```python
from build123d import *

# Parameters (mm, degrees)
F0_R     = 775
F0_R_2   = 16.5
F0_R_3   = 475
F1_DEPTH = 160
F3_DEPTH = 160


with BuildPart() as f1:
    # F0 (on Front) → F1 (new body)
    with BuildSketch(Plane.XZ):
        Circle(F0_R)
        with Locations((-389.681126, -488.644677)):
            Circle(F0_R_2, mode=Mode.SUBTRACT)
        with Locations((-488.644677, -389.681126)):
            Circle(F0_R_2, mode=Mode.SUBTRACT)
        with Locations((-441.941738, -441.941738)):
            Circle(F0_R_2, mode=Mode.SUBTRACT)
        with Locations((-206.424414, -589.927081)):
            Circle(F0_R_2, mode=Mode.SUBTRACT)
        with Locations((-139.075584, -609.329945)):
            Circle(F0_R_2, mode=Mode.SUBTRACT)
        with Locations((-69.977798, -621.070131)):
            Circle(F0_R_2, mode=Mode.SUBTRACT)
        with Locations((-332.520048, -529.202625)):
            Circle(F0_R_2, mode=Mode.SUBTRACT)
        with Locations((-271.177337, -563.105542)):
            Circle(F0_R_2, mode=Mode.SUBTRACT)
        with Locations((-589.927081, -206.424414)):
            Circle(F0_R_2, mode=Mode.SUBTRACT)
        with Locations((-529.202625, -332.520048)):
            Circle(F0_R_2, mode=Mode.SUBTRACT)
        with Locations((-563.105542, -271.177337)):
            Circle(F0_R_2, mode=Mode.SUBTRACT)
        with Locations((-609.329945, -139.075584)):
            Circle(F0_R_2, mode=Mode.SUBTRACT)
        with Locations((-621.070131, -69.977798)):
            Circle(F0_R_2, mode=Mode.SUBTRACT)
        with Locations((0, -625)):
            Circle(F0_R_2, mode=Mode.SUBTRACT)
        with Locations((69.977798, -621.070131)):
            Circle(F0_R_2, mode=Mode.SUBTRACT)
        with Locations((139.075584, -609.329945)):
            Circle(F0_R_2, mode=Mode.SUBTRACT)
        with Locations((206.424414, -589.927081)):
            Circle(F0_R_2, mode=Mode.SUBTRACT)
        with Locations((271.177337, -563.105542)):
            Circle(F0_R_2, mode=Mode.SUBTRACT)
        with Locations((332.520048, -529.202625)):
            Circle(F0_R_2, mode=Mode.SUBTRACT)
        with Locations((389.681126, -488.644677)):
            Circle(F0_R_2, mode=Mode.SUBTRACT)
        with Locations((441.941738, -441.941738)):
            Circle(F0_R_2, mode=Mode.SUBTRACT)
        with Locations((488.644677, -389.681126)):
            Circle(F0_R_2, mode=Mode.SUBTRACT)
        with Locations((529.202625, -332.520048)):
            Circle(F0_R_2, mode=Mode.SUBTRACT)
        with Locations((563.105542, -271.177337)):
            Circle(F0_R_2, mode=Mode.SUBTRACT)
        with Locations((589.927081, -206.424414)):
            Circle(F0_R_2, mode=Mode.SUBTRACT)
        with Locations((609.329945, -139.075584)):
            Circle(F0_R_2, mode=Mode.SUBTRACT)
        with Locations((621.070131, -69.977798)):
            Circle(F0_R_2, mode=Mode.SUBTRACT)
        with Locations((-625, 0)):
            Circle(F0_R_2, mode=Mode.SUBTRACT)
        with Locations((-621.070131, 69.977798)):
            Circle(F0_R_2, mode=Mode.SUBTRACT)
        with Locations((-609.329945, 139.075584)):
            Circle(F0_R_2, mode=Mode.SUBTRACT)
        with Locations((-589.927081, 206.424414)):
            Circle(F0_R_2, mode=Mode.SUBTRACT)
        with Locations((-563.105542, 271.177337)):
            Circle(F0_R_2, mode=Mode.SUBTRACT)
        with Locations((-529.202625, 332.520048)):
            Circle(F0_R_2, mode=Mode.SUBTRACT)
        with Locations((-488.644677, 389.681126)):
            Circle(F0_R_2, mode=Mode.SUBTRACT)
        with Locations((-441.941738, 441.941738)):
            Circle(F0_R_2, mode=Mode.SUBTRACT)
        with Locations((-389.681126, 488.644677)):
            Circle(F0_R_2, mode=Mode.SUBTRACT)
        with Locations((-332.520048, 529.202625)):
            Circle(F0_R_2, mode=Mode.SUBTRACT)
        with Locations((-271.177337, 563.105542)):
            Circle(F0_R_2, mode=Mode.SUBTRACT)
        with Locations((-206.424414, 589.927081)):
            Circle(F0_R_2, mode=Mode.SUBTRACT)
        with Locations((-139.075584, 609.329945)):
            Circle(F0_R_2, mode=Mode.SUBTRACT)
        with Locations((-69.977798, 621.070131)):
            Circle(F0_R_2, mode=Mode.SUBTRACT)
        Circle(F0_R_3, mode=Mode.SUBTRACT)
        with Locations((625, 0)):
            Circle(F0_R_2, mode=Mode.SUBTRACT)
        with Locations((621.070131, 69.977798)):
            Circle(F0_R_2, mode=Mode.SUBTRACT)
        with Locations((609.329945, 139.075584)):
            Circle(F0_R_2, mode=Mode.SUBTRACT)
        with Locations((563.105542, 271.177337)):
            Circle(F0_R_2, mode=Mode.SUBTRACT)
        with Locations((529.202625, 332.520048)):
            Circle(F0_R_2, mode=Mode.SUBTRACT)
        with Locations((589.927081, 206.424414)):
            Circle(F0_R_2, mode=Mode.SUBTRACT)
        with Locations((271.177337, 563.105542)):
            Circle(F0_R_2, mode=Mode.SUBTRACT)
        with Locations((332.520048, 529.202625)):
            Circle(F0_R_2, mode=Mode.SUBTRACT)
        with Locations((0, 625)):
            Circle(F0_R_2, mode=Mode.SUBTRACT)
        with Locations((69.977798, 621.070131)):
            Circle(F0_R_2, mode=Mode.SUBTRACT)
        with Locations((139.075584, 609.329945)):
            Circle(F0_R_2, mode=Mode.SUBTRACT)
        with Locations((206.424414, 589.927081)):
            Circle(F0_R_2, mode=Mode.SUBTRACT)
        with Locations((441.941738, 441.941738)):
            Circle(F0_R_2, mode=Mode.SUBTRACT)
        with Locations((488.644677, 389.681126)):
            Circle(F0_R_2, mode=Mode.SUBTRACT)
        with Locations((389.681126, 488.644677)):
            Circle(F0_R_2, mode=Mode.SUBTRACT)
    extrude(amount=F1_DEPTH)


with BuildPart() as f3:
    # F2 (on Front) → F3 (new body)
    with BuildSketch(Plane.XZ):
        Polygon((78.170491, 1393.816872), (0, 0), (1136.468839, 1015.763554), align=None)
    extrude(amount=F3_DEPTH)


with BuildPart() as f1_1:
    add(f1.part)

    # F4: intersect F3
    add(f3.part, mode=Mode.INTERSECT)


solid = f1_1.part
```
Here's how the part is built. I have some questions about the finished solid (model axes, mm). Coordinates: 2 decimals unless noted, no trailing zeros. Write each loop counter-clockwise with the first axis right and the second up, starting at its lowest first coordinate (ties: lowest second). Pieces come first, ordered by that corner, then holes. Notation, with made-up numbers: (0, 51) - (38, 51) arc R38 ccw to (38, 89) - close; hole circle Ø7 at (29.25, 17.25). An arc over 180 degrees is marked (long way). One line per item, written item: value.
1) I need wall thicknesses on line 1 along Z through (x, y) = (77.5, -52); line 2 along X through (y, z) = (-142, 478.5); line 3 along Z through (x, y) = (75.5, -11.5). Which ranges of each line are inside material? Lowest first, please.
Model answer:
line 1: z = 468.63 to 606.38, 635.76 to 771.12
line 2: x = 26.84 to 376.67, 402.69 to 535.36
line 3: z = 468.96 to 605.52, 636.62 to 771.31
2) Suppose I cut it at D-D on z = 685. Write out the boundary of the cut face in (x, y), and give its area (3 significant figures).
Model answer:
outline: (38.42, -160) - (362.49, -160) - (362.49, 0) - (38.42, 0) - close
area: 51,900 mm²
3) We'd pull the mould along X, two halves only. Please class faces 1 (the cylindrical face through (208.413, -78.88, 426.836)), 2 (the cylindrical face through (398.55, -78.88, 502.56)), 3 (the flat face through (298, 0, 548)), 4 (the cylindrical face through (267.6, -78.9, 547)): pulls with the +X half, pulls with the -X half, needs draft (parallel to the pull), parting line crosses it, or undercut.
Model answer:
face 1: pulls with the -X half
face 2: undercut
face 3: needs draft
face 4: undercut
4) Suppose I cut it at B-B on y = -130. Write out the boundary of the cut face in (x, z), and give its area (3 significant figures).
Model answer:
outline: (26.6, 474.25) arc R475 cw to (354.16, 316.54) - (577.83, 516.46) arc R775 ccw to (43.4, 773.78) - close; hole circle Ø33 at (69.98, 621.07); hole circle Ø33 at (139.08, 609.33); hole circle Ø33 at (206.42, 589.93); hole circle Ø33 at (271.18, 563.11); hole circle Ø33 at (332.52, 529.2); hole circle Ø33 at (389.68, 488.64); hole circle Ø33 at (441.94, 441.94)
area: 141,000 mm²
5) Suppose I cut it at A-A on x = 451. Write out the boundary of the cut face in (y, z), and give its area (3 significant figures).
Model answer:
outline: (-160, 403.1) - (0, 403.1) - (0, 428.15) - (-160, 428.15) - close; (-160, 455.73) - (0, 455.73) - (0, 630.26) - (-160, 630.26) - close
area: 31,900 mm²
6) Suppose I cut it at C-C on x = 200.5. Write out the boundary of the cut face in (y, z), and give its area (3 significant figures).
Model answer:
outline: (-160, 430.61) - (0, 430.61) - (0, 574.53) - (-160, 574.53) - close; (-160, 605.33) - (0, 605.33) - (0, 748.62) - (-160, 748.62) - close
area: 46,000 mm²
7) I'm going to push flat-ended pins straight in: P1, Ø3, axis at y = -116.5, z = 580.5, coming from the +X side; P2, Ø10, axis at y = -132, z = 367, coming from the +X side; P3, Ø8, axis at x = 181, y = -104.5, coming from the +Z side. Where does each tip first touch, or does it pass through?
Model answer:
P1: stops at x = 515.15
P2: stops at x = 416.21
P3: stops at z = 754.52
